Geometry check sheet. Reference: the model listing, model coordinates, mm. A direction names the side the tool comes from. Give positions to 0.01 mm unless a question says otherwise; leave off trailing zeros. Write each loop counter-clockwise with the first axis right and the second up, starting at its lowest first coordinate (ties: lowest second). Pieces come first, ordered by that corner, then holes. Notation, with made-up numbers: (22, 14) - (48, 14) arc R31 ccw to (48, 40) - close; hole circle Ø6 at (37, 10). An arc over 180 degrees is marked (long way). Use a Markdown table: item, result.
```python
from build123d import *

# Parameters (mm, degrees)
F2_DEPTH = 25.4
F3_DEPTH = 25.4


with BuildPart() as f2:
    # F0 (on Front) → F2 (new body)
    with BuildSketch(Plane.XZ):
        Polygon((0, 6.35), (0, 0), (25.4, 0), (25.4, 6.35), (16.920075, 6.35), align=None)
        Polygon((0, 19.05), (0, 6.35), (16.920075, 6.35), (16.920075, 12.7), (8.440151, 19.05), align=None)
    extrude(amount=-F2_DEPTH)

    # F1 (on Right) → F3 (join)
    with BuildSketch(Plane.YZ):
        Polygon((0, 6.35), (0, 0), (38.1, 0), (38.1, 6.35), (25.4, 6.35), (12.7, 6.35), align=None)
        Polygon((25.4, 6.35), (38.1, 6.35), (38.1, 25.4), (25.4, 25.4), (25.4, 19.05), (12.7, 19.05), (12.7, 12.7), (25.4, 12.7), align=None)
    extrude(amount=F3_DEPTH)


solid = f2.part
```
1) Section check D-D on x = 6. Record the boundary of the cut face in (y, z), then the cut area to 3 significant figures.
Working result:
| item | result |
|---|---|
| outline | (0, 0) - (38.1, 0) - (38.1, 25.4) - (25.4, 25.4) - (25.4, 19.05) - (0, 19.05) - close |
| area | 806 mm² |
2) Material ranges on L1, parallel to Z at x = 24.25, y = 24.5; L2, parallel to Y at x = 11.25, z = 17.75; L3, parallel to Z at x = 2.25, y = 6, recorded low to high. Write a range as from..to.
Working result:
| item | result |
|---|---|
| L1 | z = 0..6.35, 12.7..19.05 |
| L2 | y = 12.7..38.1 |
| L3 | z = 0..19.05 |
3) Section check C-C on z = 22. Record the boundary of the cut face in (x, y), then the cut area to 3 significant figures.
Working result:
| item | result |
|---|---|
| outline | (0, 25.4) - (25.4, 25.4) - (25.4, 38.1) - (0, 38.1) - close |
| area | 323 mm² |
4) Mould release check, pull along Z, two halves, no side actions. Record for faces 1 (the flat face through (13, 19, 0)), 2 (the flat face through (10, 0, 8)), 3 (the flat face through (21, 19, 12.7)): pulls with the +Z half, pulls with the -Z half, needs draft (parallel to the pull), parting line crosses it, or undercut.
Working result:
| item | result |
|---|---|
| face 1 | pulls with the -Z half |
| face 2 | needs draft |
| face 3 | undercut |
5) Set-up check for faces 4 (the flat face through (25.4, 27, 10)), 5 (the flat face through (16.92, 13, 9)), 6 (the flat face through (13, 38.1, 13)), 7 (the flat face through (12.74, 6.26, 15.83)), 8 (the flat face through (13, 25.4, 22)): record each of +Z, -Z, +X, -X, +Y, -Y from which the full face is reachable in a straight line by a thin tool's end or side.
Working result:
| item | result |
|---|---|
| face 4 | +Z, -Z, +X, +Y, -Y |
| face 5 | +X, -Y |
| face 6 | +Z, -Z, +X, -X, +Y |
| face 7 | +Z, +X, -Y |
| face 8 | +Z, +X, -X, -Y |
6) Depth check by flat-ended pin: P1, Ø3, axis at x = 7, y = 12.5, coming from the +Z side; P2, Ø3, axis at x = 18.5, z = 22.5, coming from the -Y side; P3, Ø2, axis at y = 11.5, z = 14.5, coming from the +X side. Enter the tip coordinate at first touch or a pass-through.
Working result:
| item | result |
|---|---|
| P1 | stops at z = 19.05 |
| P2 | stops at y = 25.4 |
| P3 | stops at x = 15.85 |
7) Section check A-A on x = 23.75. Record the boundary of the cut face in (y, z), then the cut area to 3 significant figures.
Working result:
| item | result |
|---|---|
| outline | (0, 0) - (38.1, 0) - (38.1, 25.4) - (25.4, 25.4) - (25.4, 19.05) - (12.7, 19.05) - (12.7, 12.7) - (25.4, 12.7) - (25.4, 6.35) - (0, 6.35) - close |
| area | 565 mm² |
8) Section check B-B on y = 3.5. Record the boundary of the cut face in (x, z), then the cut area to 3 significant figures.
Working result:
| item | result |
|---|---|
| outline | (0, 0) - (25.4, 0) - (25.4, 6.35) - (16.92, 6.35) - (16.92, 12.7) - (8.44, 19.05) - (0, 19.05) - close |
| area | 349 mm² |
